from build123d import *

# Parameters (mm, degrees)
EXTRUDE_1_DEPTH     = 2
CUT_EXTRUDE_2_DEPTH = 2.2


with BuildPart() as part:
    # ｽｹｯﾁ1 → ﾎﾞｽ - 押し出し1 (new body)
    with BuildSketch(Plane(origin=(0, 0, 0), x_dir=(1, 0, 0), z_dir=(0, 1, 0))):
        with BuildLine():
            Line((2.65, 4.705050478), (2.65, 2.65))
            Line((2.65, 2.65), (4.705050478, 2.65))
            ThreePointArc((4.705050478, 2.65), (5.4, 0), (4.705050478, -2.65))
            Line((4.705050478, -2.65), (2.65, -2.65))
            Line((2.65, -2.65), (2.65, -4.705050478))
            ThreePointArc((2.65, -4.705050478), (0, -5.4), (-2.65, -4.705050478))
            Line((-2.65, -4.705050478), (-2.65, -2.65))
            Line((-2.65, -2.65), (-4.705050478, -2.65))
            ThreePointArc((-4.705050478, -2.65), (-5.4, 0), (-4.705050478, 2.65))
            Line((-4.705050478, 2.65), (-2.65, 2.65))
            Line((-2.65, 2.65), (-2.65, 4.705050478))
            ThreePointArc((-2.65, 4.705050478), (0, 5.4), (2.65, 4.705050478))
        make_face()
    extrude(amount=EXTRUDE_1_DEPTH)

    # ｽｹｯﾁ4 → ｶｯﾄ - 押し出し2 (cut)
    with BuildSketch(Plane(origin=(0, 2, 0), x_dir=(1, 0, 0), z_dir=(0, 1, 0))):
        Polygon((0, 1.6), (0.437016815, 2.056002469), (0.650778629, 1.461672732), (1.235486269, 1.700500964), (1.189031721, 1.07060897), (1.820328922, 1.050967393), (1.521690426, 0.494427191), (2.090420168, 0.219712013), (1.591235033, -0.167245541), (1.999058776, -0.64953357), (1.385640646, -0.8), (1.56204196, -1.406468898), (0.940456404, -1.294427191), (0.854933899, -1.920212977), (0.332658705, -1.565036161), (0, -2.101934787), (-0.332658705, -1.565036161), (-0.854933899, -1.920212977), (-0.940456404, -1.294427191), (-1.56204196, -1.406468898), (-1.385640646, -0.8), (-1.999058776, -0.64953357), (-1.591235033, -0.167245541), (-2.090420168, 0.219712013), (-1.521690426, 0.494427191), (-1.820328922, 1.050967393), (-1.189031721, 1.07060897), (-1.235486269, 1.700500964), (-0.650778629, 1.461672732), (-0.437016815, 2.056002469), align=None)
    extrude(amount=-CUT_EXTRUDE_2_DEPTH, mode=Mode.SUBTRACT)


solid = part.part
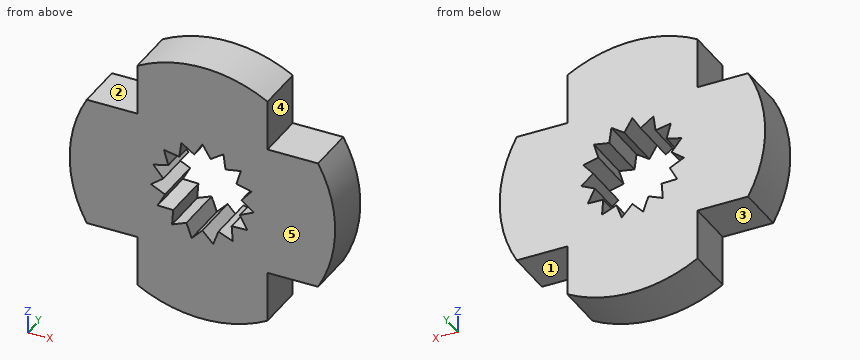
Could you check a few things on this model? Use its own coordinates, in mm. Face numbers are marked on the shaded views. A direction names the side the tool comes from. Coordinates: 2 decimals unless noted, no trailing zeros. Loops run counter-clockwise (first coordinate to the right, second up) from the corner with the lowest first, then second, coordinate; pieces in that order, holes last. Notation, with made-up numbers: (50.5, 83.25) -> (69.5, 83.25) arc R23 ccw to (69.5, 122.25) -> close; hole circle Ø8 at (32.5, 64). An arc over 180 degrees is marked (long way). Answer in a Markdown table with one row per item.
(1) Will these pins go through, and if not, where does the flat tip stop? pin 1 Ø1 at (y, z) = (1, -3.5) entering from -X; pin 2 Ø1 at (x, y) = (4, 1.5) entering from +Z.
Results found:
| item | result |
|---|---|
| pin 1 | stops at x = -2.65 |
| pin 2 | stops at z = 2.65 |
(2) If I drill on probe 1 along X at (y, z) = (0.8, 3.75), over which ranges is the centre line in solid material (lowest first)?
Results found:
| item | result |
|---|---|
| probe 1 | x = -2.65 to 2.65 |
(3) Imagine slicing it at A-A (z = 4). List the corners of the cut face in (x, y) for me, plus the area to 3 significant figures.
Results found:
| item | result |
|---|---|
| outline | (-2.65, 0) -> (2.65, 0) -> (2.65, 2) -> (-2.65, 2) -> close |
| area | 10.6 mm^2 |
(4) For the marked faces 1, 2, 3, 4 and 5, which set-ups out of +Z, -Z, +X, -X, +Y, -Y let a thin tool reach every point of the face, with its end or its side?
Results found:
| item | result |
|---|---|
| face 1 | -Z, +X, +Y, -Y |
| face 2 | +Z, -X, +Y, -Y |
| face 3 | -Z, -X, +Y, -Y |
| face 4 | +Z, +X, +Y, -Y |
| face 5 | +Z, -Z, +X, -X, -Y |
(5) Imagine slicing it at B-B (x = 2.5). List the corners of the cut face in (y, z) for me.
Results found:
| item | result |
|---|---|
| outline | (0, -4.79) -> (2, -4.79) -> (2, 4.79) -> (0, 4.79) -> close |
